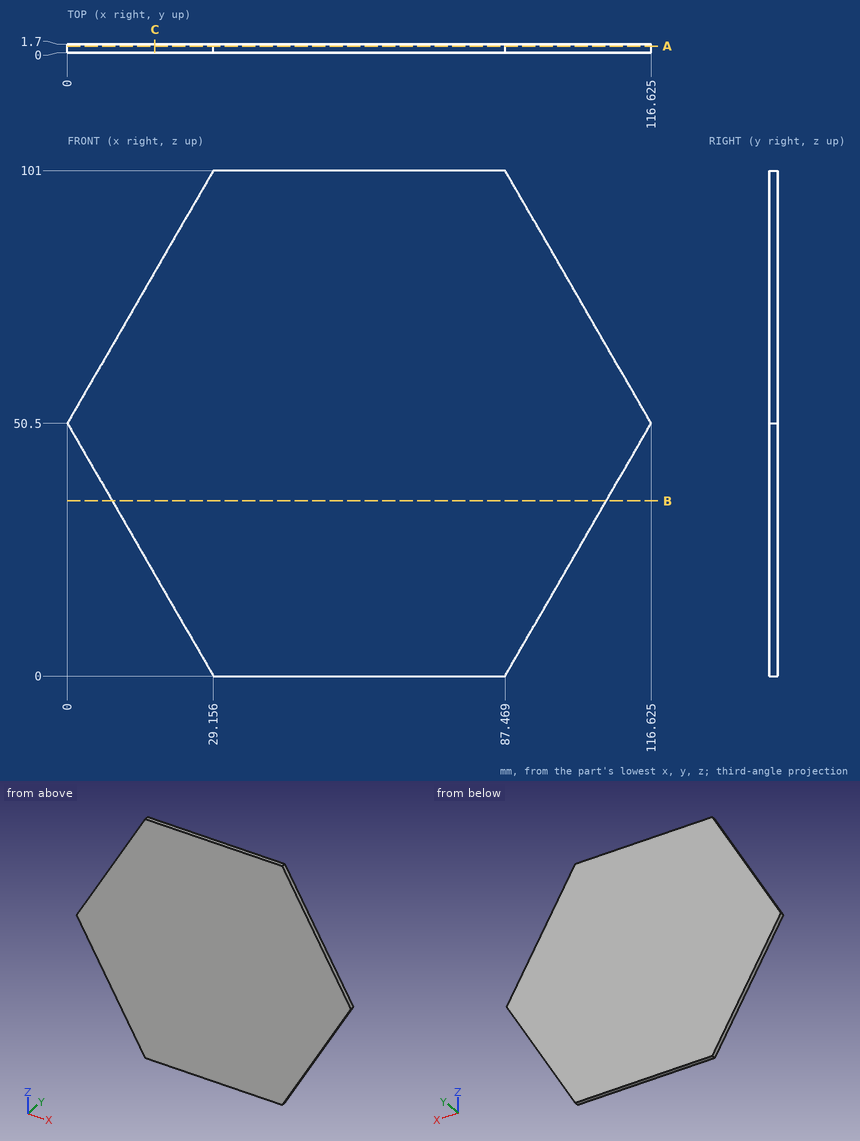
Answer from the drawing. Dimensions are ordinates in mm from the lowest x, y and z of the part. Round coordinates to 2 decimals unless told otherwise and drop trailing zeros. Loops run counter-clockwise (first coordinate to the right, second up) from the corner with the lowest first, then second, coordinate; pieces in that order, holes last. Notation, with made-up numbers: (47, 9) - (67, 9) arc R28 ccw to (67, 29) - close; hole circle Ø9 at (-1, 41). An arc over 180 degrees is marked (long way). One line per item, written item: value.
Q1. Straight lines are drawn through the part: probe 1 along Z at (x, y) = (104.5, 0.7); probe 2 along X at (y, z) = (0.95, 32.5); probe 3 along Z at (x, y) = (5, 0.2). For each, find the intervals that lie inside material, in ascending order.
Check values:
probe 1: 29.5 to 71.5
probe 2: 10.39 to 106.23
probe 3: 41.84 to 59.16
Q2. Find section A-A on y = 1.25. Give the vertices of the cut face in (x, z) (1 decimal), and give its area (3 significant figures).
Check values:
outline: (0, 50.5) - (29.2, 0) - (87.5, 0) - (116.6, 50.5) - (87.5, 101) - (29.2, 101) - close
area: 8,830 mm2
Q3. Find section B-B on z = 35. Give the vertices of the cut face in (x, y).
Check values:
outline: (8.95, 0) - (107.68, 0) - (107.68, 1.7) - (8.95, 1.7) - close
Q4. Find section C-C on x = 17.5. Give the vertices of the cut face in (y, z).
Check values:
outline: (0, 20.19) - (1.7, 20.19) - (1.7, 80.81) - (0, 80.81) - close
